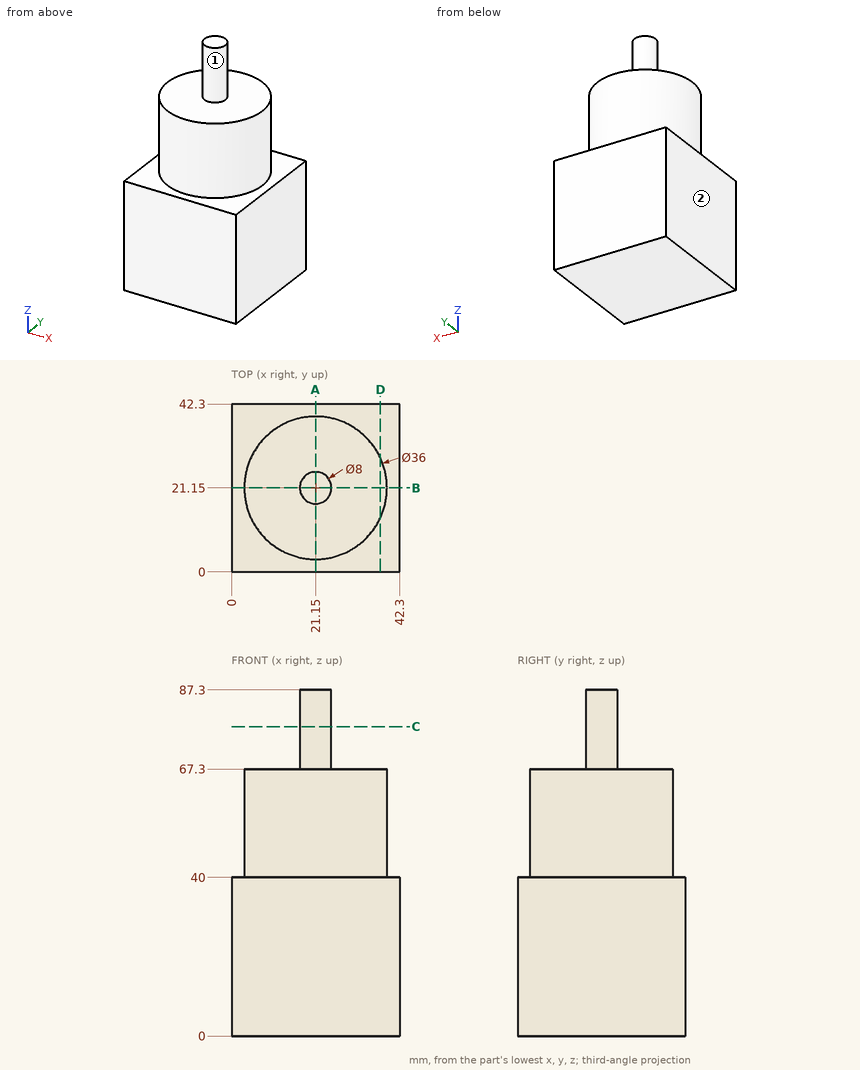
The figure shows three views and two pictorial views of one solid part (mm, origin at its lowest corner). Answer the questions. A direction names the side the tool comes from. Give positions to 0.01 mm unless a question says otherwise; leave off trailing zeros. Write each loop counter-clockwise with the first axis right and the second up, starting at its lowest first coordinate (ties: lowest second). Pieces come first, ordered by that corner, then holes. Notation, with made-up numbers: (13.5, -6) -> (63.5, -6) arc R27 ccw to (63.5, 23) -> close; hole circle Ø11 at (75.5, 11.5). An arc over 180 degrees is marked (long way). Answer as a JSON object with one key per item and string values.
1) Section D-D on x = 37.5 is taken. Write down the section's boundary in (y, z).
Findings below:
{"outline": "(0, 0) -> (42.3, 0) -> (42.3, 40) -> (28.68, 40) -> (28.68, 67.3) -> (13.62, 67.3) -> (13.62, 40) -> (0, 40) -> close"}
2) A tool of negligible diameter and unlimited length cuts with its end or side. For the marked faces 1 and 2, from which of +Z, -Z, +X, -X, +Y, -Y can it reach the whole face along a straight path? Write none if from no direction.
Findings below:
{"face 1": "+Z", "face 2": "+Z, -Z, -X, +Y, -Y"}
3) Straight lines are drawn through the part: probe 1 along Z at (x, y) = (25.5, 37); probe 2 along Z at (x, y) = (38.5, 14.5); probe 3 along X at (y, z) = (16, 50). For each, find the intervals that lie inside material, in ascending order. Write a range as from..to.
Findings below:
{"probe 1": "z = 0..67.3", "probe 2": "z = 0..40", "probe 3": "x = 3.9..38.4"}
4) Section A-A on x = 21.15 is taken. Write down the section's boundary in (y, z).
Findings below:
{"outline": "(0, 0) -> (42.3, 0) -> (42.3, 40) -> (39.15, 40) -> (39.15, 67.3) -> (25.15, 67.3) -> (25.15, 87.3) -> (17.15, 87.3) -> (17.15, 67.3) -> (3.15, 67.3) -> (3.15, 40) -> (0, 40) -> close"}
5) Section C-C on z = 78 is taken. Write down the section's boundary in (x, y).
Findings below:
{"outline": "circle Ø8 at (21.15, 21.15)"}
6) Flat-ended cylindrical pins translate along their axes: pin 1 Ø4 at (x, y) = (10.5, 31.5) entering from -Z; pin 2 Ø5 at (y, z) = (23, 49.5) entering from -X; pin 3 Ø1 at (x, z) = (13.5, 61.5) entering from -Y; pin 4 Ø1 at (x, y) = (7.5, 21) entering from +Z. Find the tip coordinate at first contact, or state that the pin passes through.
Findings below:
{"pin 1": "stops at z = 0", "pin 2": "stops at x = 3.15", "pin 3": "stops at y = 4.63", "pin 4": "stops at z = 67.3"}
